Check sheet for the drawn part. Datum: minimum x, y, z corner. Units: mm. Coordinates: 2 decimals unless noted, no trailing zeros. Loops run counter-clockwise (first coordinate to the right, second up) from the corner with the lowest first, then second, coordinate; pieces in that order, holes last. Notation, with made-up numbers: M 65,-11.75 L 121,-11.75 A13 ccw 121,1.25 Z; hole C 21.25,45.5 d8. An arc over 180 degrees is marked long. Answer in a Markdown table with one row per item. Add a question column.
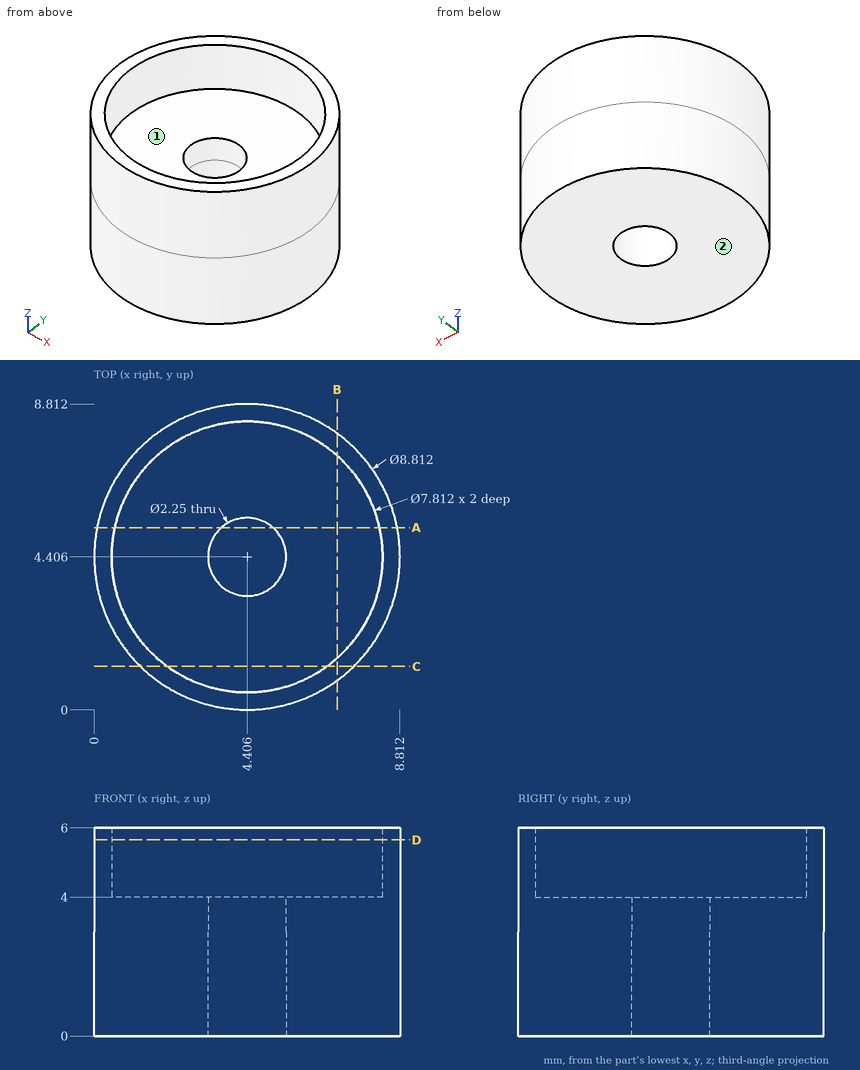
Q1. Cross-section at A-A (y = 5.25). Record the cut outline in (x, z).
Q2. Mould release check, pull along Y, two halves, no side actions. Record for the marked faces 1 and 2: released by +Y, released by -Y, zero draft, split by the parting line, or undercut.
Q3. Thickness scan on L1, parallel to X at y = 7.75, z = 4.85 (1 decimal); L2, parallel to Y at x = 4.75, z = 2.75 (1 decimal). Record the ranges inside material, lowest first.
Q4. Cross-section at D-D (z = 5.65). Record the cut outline in (x, y).
Q5. Cross-section at C-C (y = 1.25). Record the cut outline in (x, z) (1 decimal).
Q6. Cross-section at B-B (x = 7). Record the cut outline in (y, z) (1 decimal).
Q7. Go/stop test with flat-tipped pins: pin 1 (3.5 mm diameter, centred on x = 4.41, y = 4.41, fed in from +Z); pin 2 (2 mm diameter, centred on x = 4.41, y = 4.41, fed in from +Z) (3 decimals). Record where each tip stops, or that it passes through.
Answer key:
| question | item | result |
|---|---|---|
| 1 | outline | M 0.08,0 L 3.66,0 L 3.66,4 L 0.59,4 L 0.59,6 L 0.08,6 Z; M 5.15,0 L 8.73,0 L 8.73,6 L 8.22,6 L 8.22,4 L 5.15,4 Z |
| 2 | face 1 | undercut |
| 2 | face 2 | zero draft |
| 3 | L1 | 1.5 to 2.4, 6.4 to 7.3 |
| 3 | L2 | 0 to 3.3, 5.5 to 8.8 |
| 4 | outline | C 4.41,4.41 d8.81; hole C 4.41,4.41 d7.81 |
| 5 | outline | M 1.3,0 L 7.5,0 L 7.5,6 L 6.7,6 L 6.7,4 L 2.1,4 L 2.1,6 L 1.3,6 Z |
| 6 | outline | M 0.8,0 L 8,0 L 8,6 L 7.3,6 L 7.3,4 L 1.5,4 L 1.5,6 L 0.8,6 Z |
| 7 | pin 1 | z = 4 |
| 7 | pin 2 | through |
